from build123d import *

# Parameters (mm, degrees)
SKETCH1_R           = 30.25
SKETCH1_R_2         = 25.25
EXTRUDE_THIN1_DEPTH = 3
SKETCH2_R           = 1.65
CUT_EXTRUDE3_DEPTH  = 10
BOSS_EXTRUDE1_DEPTH = 3


with BuildPart() as part:
    # Sketch1 → Extrude-Thin1 (new body)
    with BuildSketch(Plane(origin=(0, 0, 0), x_dir=(1, 0, 0), z_dir=(0, 1, 0))):
        Circle(SKETCH1_R)
        Circle(SKETCH1_R_2, mode=Mode.SUBTRACT)
    extrude(amount=-EXTRUDE_THIN1_DEPTH)

    # Sketch2 → Cut-Extrude3 (cut)
    with BuildSketch(Plane(origin=(0, 0, 0), x_dir=(1, 0, 0), z_dir=(0, 1, 0))):
        with Locations((0, 27.5)):
            Circle(SKETCH2_R)
        with Locations((23.815698604, -13.75)):
            Circle(SKETCH2_R)
        with Locations((-23.815698604, -13.75)):
            Circle(SKETCH2_R)
    extrude(amount=-CUT_EXTRUDE3_DEPTH, mode=Mode.SUBTRACT)

    # Sketch5 → Boss-Extrude1 (add)
    with BuildSketch(Plane.XZ.offset(3)):
        with BuildLine():
            Line((0, 45.25), (0, 30.25))
            ThreePointArc((0, 30.25), (4.209986304, 29.955609079), (8.338030013, 29.078166302))
            Line((8.338030013, 29.078166302), (12.472590351, 43.497091741))
            ThreePointArc((12.472590351, 43.497091741), (6.297582818, 44.809630111), (0, 45.25))
        make_face()
        with BuildLine():
            Line((31.996581849, 31.996581849), (21.389980131, 21.389980131))
            ThreePointArc((21.389980131, 21.389980131), (24.158724179, 18.20490445), (26.457246141, 14.665491012))
            Line((26.457246141, 14.665491012), (39.576541748, 21.937635316))
            ThreePointArc((39.576541748, 21.937635316), (36.13825683, 27.232129798), (31.996581849, 31.996581849))
        make_face()
        with BuildLine():
            Line((45.25, 0), (30.25, 0))
            ThreePointArc((30.25, 0), (29.955609079, -4.209986304), (29.078166302, -8.338030013))
            Line((29.078166302, -8.338030013), (43.497091741, -12.472590351))
            ThreePointArc((43.497091741, -12.472590351), (44.809630111, -6.297582818), (45.25, 0))
        make_face()
        with BuildLine():
            Line((31.996581849, -31.996581849), (21.389980131, -21.389980131))
            ThreePointArc((21.389980131, -21.389980131), (18.20490445, -24.158724179), (14.665491012, -26.457246141))
            Line((14.665491012, -26.457246141), (21.937635316, -39.576541748))
            ThreePointArc((21.937635316, -39.576541748), (27.232129798, -36.13825683), (31.996581849, -31.996581849))
        make_face()
        with BuildLine():
            Line((0, -45.25), (0, -30.25))
            ThreePointArc((0, -30.25), (-4.209986304, -29.955609079), (-8.338030013, -29.078166302))
            Line((-8.338030013, -29.078166302), (-12.472590351, -43.497091741))
            ThreePointArc((-12.472590351, -43.497091741), (-6.297582818, -44.809630111), (0, -45.25))
        make_face()
        with BuildLine():
            Line((-31.996581849, -31.996581849), (-21.389980131, -21.389980131))
            ThreePointArc((-21.389980131, -21.389980131), (-24.158724179, -18.20490445), (-26.457246141, -14.665491012))
            Line((-26.457246141, -14.665491012), (-39.576541748, -21.937635316))
            ThreePointArc((-39.576541748, -21.937635316), (-36.13825683, -27.232129798), (-31.996581849, -31.996581849))
        make_face()
        with BuildLine():
            Line((-45.25, 0), (-30.25, 0))
            ThreePointArc((-30.25, 0), (-29.955609079, 4.209986304), (-29.078166302, 8.338030013))
            Line((-29.078166302, 8.338030013), (-43.497091741, 12.472590351))
            ThreePointArc((-43.497091741, 12.472590351), (-44.809630111, 6.297582818), (-45.25, 0))
        make_face()
        with BuildLine():
            Line((-31.996581849, 31.996581849), (-21.389980131, 21.389980131))
            ThreePointArc((-21.389980131, 21.389980131), (-18.20490445, 24.158724179), (-14.665491012, 26.457246141))
            Line((-14.665491012, 26.457246141), (-21.937635316, 39.576541748))
            ThreePointArc((-21.937635316, 39.576541748), (-27.232129798, 36.13825683), (-31.996581849, 31.996581849))
        make_face()
    extrude(amount=-BOSS_EXTRUDE1_DEPTH)


solid = part.part
Model file for the job. Use its own axes, mm. A direction names the side the tool comes from. Give positions to 0.01 mm unless a question says otherwise; leave off trailing zeros. Order: outer loops, then holes, each group sorted by start corner. A loop starts at its lowest first (then second) coordinate and runs counter-clockwise, first axis right, second up. Notation, with made-up numbers: (10, 31.5) - (66, 31.5) arc R25 cw to (66, 64.5) - close; hole circle Ø3 at (20, 76.5). An arc over 180 degrees is marked (long way). Return JSON: item names as keys, results as strings.
1) Pull direction Z, two halves, no side cores. Call faces 1 (the cylindrical face through (27.16, -1.52, -36.19)), 2 (the flat face through (-36.187, -1.521, 10.376)), 3 (the flat face through (0, -2, -38)), 4 (the cylindrical face through (-26.12, -1.48, 15.26)): pulls with the +Z half, pulls with the -Z half, needs draft (parallel to the pull), parting line crosses it, or undercut.
Geometry says:
{"face 1": "pulls with the -Z half", "face 2": "undercut", "face 3": "needs draft", "face 4": "undercut"}
2) Cut at B-B, the plane x = -10.5. Give the cut face in (y, z).
Geometry says:
{"outline": "(-3, -44.01) - (0, -44.01) - (0, -36.62) - (-3, -36.62) - close; (-3, -28.37) - (0, -28.37) - (0, -22.96) - (-3, -22.96) - close; (-3, 22.96) - (0, 22.96) - (0, 28.37) - (-3, 28.37) - close"}
3) Probe line 1 (X direction, y = -0.85, z = -27.5); line 2 (Z direction, x = -22, y = -1.9); line 3 (X direction, y = -0.6, z = 13.75). List the from-to ranges inside material, lowest first. Write a range as from..to.
Geometry says:
{"line 1": "-35.93..-27.5, -12.6..-1.65, 1.65..12.6, 15.24..27.5", "line 2": "-22..-12.39, 12.39..20.76, 22..39.54", "line 3": "-26.94..-25.47, -22.17..-21.18, 21.18..22.17, 25.47..26.94"}
4) Cut at C-C, the plane x = 16.5. Give the cut face in (y, z), plus the area to 3 significant figures.
Geometry says:
{"outline": "(-3, -29.77) - (0, -29.77) - (0, -19.11) - (-3, -19.11) - close; (-3, 19.11) - (0, 19.11) - (0, 25.35) - (-3, 25.35) - close", "area": "50.7 mm²"}
5) Flat gauge pins, fed straight in: P1, Ø3, axis at x = 0, z = -27.5, coming from the -Y side; P2, Ø1, axis at y = -1, z = -21.5, coming from the -X side; P3, Ø1.5, axis at x = 34, y = -1.5, coming from the +Z side. Where does each tip first touch, or does it go through?
Geometry says:
{"P1": "through", "P2": "x = -39.58", "P3": "z = 30.69"}
6) Cut at A-A, the plane z = -20. Give the cut face in (x, y), plus the area to 3 significant figures.
Geometry says:
{"outline": "(-36.08, -3) - (-15.41, -3) - (-15.41, 0) - (-36.08, 0) - close; (15.41, -3) - (22.69, -3) - (22.69, 0) - (15.41, 0) - close", "area": "83.8 mm²"}
7) 3-axis set-ups, long thin cutter, end or side, ignore diameter. For faces 5 (the flat face through (-38, -2, 0)), 6 (the cylindrical face through (-36.19, -1.52, -27.16)), 7 (the cylindrical face through (26.12, -1.48, -15.26)), 8 (the cylindrical face through (29.26, -1.48, 7.68)), 9 (the cylindrical face through (-7.68, -1.48, 29.26)): which of +Z, -Z, +X, -X, +Y, -Y reach the whole face in a straight line?
Geometry says:
{"face 5": "-X, +Y, -Y", "face 6": "-Z, -X, +Y, -Y", "face 7": "+Y, -Y", "face 8": "+X, +Y, -Y", "face 9": "+Z, +Y, -Y"}
8) Cut at D-D, the plane y = -0.95. Count the separate pieces of the cut face and the enclosed holes in it, plus the area to 3 significant figures.
Geometry says:
{"separate pieces": "1", "enclosed holes": "4", "area": "2,110 mm²"}
